The listing builds one solid part. Answer for the finished solid, in the listing's coordinates (mm). Give positions to 0.01 mm unless a question says otherwise; leave off trailing zeros. Loops run counter-clockwise (first coordinate to the right, second up) from the corner with the lowest first, then second, coordinate; pieces in that order, holes last. Notation, with made-up numbers: (-33, 66.5) - (10, 66.5) arc R20 cw to (10, 94.5) - close; hole circle Ø2 at (31.25, 27.25). An arc over 180 degrees is marked (long way). Answer in a Markdown table with one row per item. Add a question column.
```python
from build123d import *

# Parameters (mm, degrees)
SKETCH1_W               = 82.55
SKETCH1_H               = 76.2
SKETCH1_R               = 3.175
BOSS_EXTRUDE1_DEPTH     = 3.175
F_10_CLEARANCE_HOLE1_D  = 4.9784
F_1_4_CLEARANCE_HOLE1_D = 6.5278
FILLET2_R               = 3.175


with BuildPart() as part:
    # Sketch1 → Boss-Extrude1 (new body)
    # profile 1 of 4: a face of its own
    with BuildSketch(Plane.XY):
        Rectangle(SKETCH1_W, SKETCH1_H)
        Circle(SKETCH1_R, mode=Mode.SUBTRACT)
        with Locations((28.575, 25.4)):
            Circle(SKETCH1_R, mode=Mode.SUBTRACT)
        with Locations((-28.575, 25.4)):
            Circle(SKETCH1_R, mode=Mode.SUBTRACT)
    # profile 2 of 4: a face of its own
    with BuildSketch(Plane.XY):
        with Locations((-28.575, 25.4)):
            Circle(SKETCH1_R)
    # profile 3 of 4: a face of its own
    with BuildSketch(Plane.XY):
        Circle(SKETCH1_R)
    # profile 4 of 4: a face of its own
    with BuildSketch(Plane.XY):
        with Locations((28.575, 25.4)):
            Circle(SKETCH1_R)
    extrude(amount=BOSS_EXTRUDE1_DEPTH)

    # #10 Clearance Hole1 (through all)
    with Locations(Plane.XY.offset(3.175)):
        with Locations((-28.575, 25.4), (28.575, 25.4)):
            Hole(F_10_CLEARANCE_HOLE1_D / 2)

    # 1/4 Clearance Hole1 (through all)
    with Locations(Plane.XY.offset(3.175)):
        with Locations((0, 0)):
            Hole(F_1_4_CLEARANCE_HOLE1_D / 2)

    # Fillet2
    fillet2_edges = [part.edges().sort_by_distance(p)[0] for p in [
        (-41.275, -38.1, 1.5875),
        (-41.275, 38.1, 1.5875),
        (41.275, 38.1, 1.5875),
        (41.275, -38.1, 1.5875),
    ]]
    fillet(fillet2_edges, radius=FILLET2_R)


solid = part.part
```
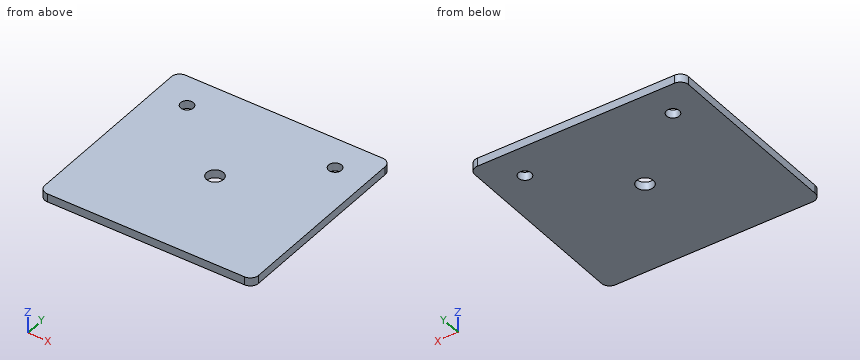
(1) A cutting plane is placed at A-A on y = 0. Determine the outline of the cut face in (x, z) (3 decimals).
(2) Find the intervals of material crossed by line 1 along Y through (x, z) = (0, 1.55); line 2 along X through (y, z) = (-3, 1.9) (3 decimals); line 3 along Y through (x, z) = (-30.5, 1.95), in increasing order. Write a range as [from, to].
(3) A cutting plane is placed at B-B on x = 0. Determine the outline of the cut face in (y, z) (3 decimals).
(4) A cutting plane is placed at C-C on y = 25.4. Determine the outline of the cut face in (x, z) (3 decimals), plus the area to 3 significant figures.
Evaluation:
| question | item | result |
|---|---|---|
| 1 | outline | (-41.275, 0) - (-3.264, 0) - (-3.264, 3.175) - (-41.275, 3.175) - close; (3.264, 0) - (41.275, 0) - (41.275, 3.175) - (3.264, 3.175) - close |
| 2 | line 1 | y = [-38.1, -3.26], [3.26, 38.1] |
| 2 | line 2 | x = [-41.275, -1.286], [1.286, 41.275] |
| 2 | line 3 | y = [-38.1, 23.82], [26.98, 38.1] |
| 3 | outline | (-38.1, 0) - (-3.264, 0) - (-3.264, 3.175) - (-38.1, 3.175) - close; (3.264, 0) - (38.1, 0) - (38.1, 3.175) - (3.264, 3.175) - close |
| 4 | outline | (-41.275, 0) - (-31.064, 0) - (-31.064, 3.175) - (-41.275, 3.175) - close; (-26.086, 0) - (26.086, 0) - (26.086, 3.175) - (-26.086, 3.175) - close; (31.064, 0) - (41.275, 0) - (41.275, 3.175) - (31.064, 3.175) - close |
| 4 | area | 230 mm² |
